```python
from build123d import *

# Parameters (mm, degrees)
SKETCH2_W            = 12
SKETCH2_H            = 29.7
BOSS_EXTRUDE1_DEPTH  = 7.8
SKETCH3_W            = 12
SKETCH3_H            = 2.2
BOSS_EXTRUDE2_DEPTH  = 5.5
CUT_EXTRUDE1_REACH   = 23.628
SKETCH4_R            = 2.35
FILLET1_R            = 1.5
FILLET1_OF_MIRROR1_R = 1.5
FILLET2_R            = 1
BOSS_EXTRUDE3_DEPTH  = 3.2
BOSS_EXTRUDE4_DEPTH  = 0.4
BOSS_EXTRUDE7_DEPTH  = 0.4
SKETCH8_R            = 1.2
BOSS_EXTRUDE6_DEPTH  = 0.2
BOSS_EXTRUDE6_TAPER  = 30
SKETCH7_R            = 2.85
BOSS_EXTRUDE5_DEPTH  = 3.4
SKETCH9_W            = 9
SKETCH9_H            = 5.6
CUT_EXTRUDE2_DEPTH   = 0.1
SKETCH10_R           = 1.1
CUT_EXTRUDE3_DEPTH   = 3
SKETCH13_R           = 4.3
BOSS_EXTRUDE8_DEPTH  = 0.4
FILLET3_R            = 0.4
CUT_EXTRUDE4_DEPTH   = 25.276789326
CIRPATTERN1_COUNT    = 23


with BuildPart() as part:
    # Sketch2 → Boss-Extrude1 (new body)
    with BuildSketch(Plane(origin=(0, 0, 0), x_dir=(1, 0, 0), z_dir=(0, 1, 0))):
        Rectangle(SKETCH2_W, SKETCH2_H)
    extrude(amount=BOSS_EXTRUDE1_DEPTH)

    # Sketch3 → Boss-Extrude2 (add)
    with BuildSketch(Plane.XY.offset(14.85)):
        with Locations((0, 3.1)):
            Rectangle(SKETCH3_W, SKETCH3_H)
    boss_extrude2 = extrude(amount=BOSS_EXTRUDE2_DEPTH)

    # Sketch4 → Cut-Extrude1 (cut, up to next)
    with BuildSketch(Plane(origin=(0, 4.2, 0), x_dir=(1, 0, 0), z_dir=(0, 1, 0)), mode=Mode.PRIVATE) as cut_extrude1_sk1:
        with Locations((0, -18.4)):
            Circle(SKETCH4_R)
    cut_extrude1_tool1 = extrude(cut_extrude1_sk1.sketch, amount=-CUT_EXTRUDE1_REACH, mode=Mode.PRIVATE) & part.part
    cut_extrude1 = cut_extrude1_tool1.solids().sort_by_distance((0, 4.2, 18.4))[0]
    add(cut_extrude1, mode=Mode.SUBTRACT)

    # Fillet1
    fillet1_edges = [part.edges().sort_by_distance(p)[0] for p in [
        (6, 3.1, 20.35),
        (-6, 3.1, 20.35),
    ]]
    fillet(fillet1_edges, radius=FILLET1_R)

    # Mirror1: Boss-Extrude2, Cut-Extrude1 across plane
    add(boss_extrude2.mirror(Plane.XY))
    add(cut_extrude1.mirror(Plane.XY), mode=Mode.SUBTRACT)

    # Fillet1 of Mirror1
    fillet1_of_mirror1_edges = [part.edges().sort_by_distance(p)[0] for p in [
        (6, 3.1, -20.35),
        (-6, 3.1, -20.35),
    ]]
    fillet(fillet1_of_mirror1_edges, radius=FILLET1_OF_MIRROR1_R)

    # Fillet2
    fillet2_edges = [part.edges().sort_by_distance(p)[0] for p in [
        (6, 1, 14.85),
        (6, 6, 14.85),
        (-6, 1, 14.85),
        (-6, 6, 14.85),
        (6, 1, -14.85),
        (6, 6, -14.85),
        (-6, 6, -14.85),
        (-6, 1, -14.85),
    ]]
    fillet(fillet2_edges, radius=FILLET2_R)

    # Sketch5 → Boss-Extrude3 (add)
    with BuildSketch(Plane(origin=(0, 7.8, 0), x_dir=(1, 0, 0), z_dir=(0, 1, 0))):
        with BuildLine():
            Line((-6, 9.155551275), (-6, 1.944448725))
            ThreePointArc((-6, 1.944448725), (-5.292143556, 0.968164496), (-4.427230154, 0.127857143))
            ThreePointArc((-4.427230154, 0.127857143), (0, -6.15), (4.427230154, 0.127857143))
            ThreePointArc((4.427230154, 0.127857143), (5.292143556, 0.968164496), (6, 1.944448725))
            Line((6, 1.944448725), (6, 9.155551275))
            ThreePointArc((6, 9.155551275), (0, 12.55), (-6, 9.155551275))
        make_face()
    extrude(amount=BOSS_EXTRUDE3_DEPTH)

    # Sketch6 → Boss-Extrude4 (add)
    with BuildSketch(Plane(origin=(0, 11, 0), x_dir=(1, 0, 0), z_dir=(0, 1, 0))):
        with BuildLine():
            Line((5.6, 2.057150161), (5.6, 9.042849839))
            ThreePointArc((5.6, 9.042849839), (0, 12.15), (-5.6, 9.042849839))
            Line((-5.6, 9.042849839), (-5.6, 2.057150161))
            ThreePointArc((-5.6, 2.057150161), (-4.856753194, 1.081001408), (-3.945673877, 0.259285714))
            ThreePointArc((-3.945673877, 0.259285714), (0, -5.75), (3.945673877, 0.259285714))
            ThreePointArc((3.945673877, 0.259285714), (4.856753194, 1.081001408), (5.6, 2.057150161))
        make_face()
    extrude(amount=BOSS_EXTRUDE4_DEPTH)

    # Sketch11 → Boss-Extrude7 (add)
    with BuildSketch(Plane(origin=(0, 7.8, 0), x_dir=(1, 0, 0), z_dir=(0, 1, 0))):
        with BuildLine():
            Line((-5.6, 13.85), (-5.6, -13.85))
            ThreePointArc((-5.6, -13.85), (-5.424264069, -14.274264069), (-5, -14.45))
            Line((-5, -14.45), (5, -14.45))
            ThreePointArc((5, -14.45), (5.424264069, -14.274264069), (5.6, -13.85))
            Line((5.6, -13.85), (5.6, 13.85))
            ThreePointArc((5.6, 13.85), (5.424264069, 14.274264069), (5, 14.45))
            Line((5, 14.45), (-5, 14.45))
            ThreePointArc((-5, 14.45), (-5.424264069, 14.274264069), (-5.6, 13.85))
        make_face()
    extrude(amount=BOSS_EXTRUDE7_DEPTH)

    # Sketch8 → Boss-Extrude6 (add)
    with BuildSketch(Plane(origin=(0, 11.4, 0), x_dir=(1, 0, 0), z_dir=(0, 1, 0))):
        with Locations((0, -1.45)):
            Circle(SKETCH8_R)
    extrude(amount=BOSS_EXTRUDE6_DEPTH, taper=BOSS_EXTRUDE6_TAPER)

    # Sketch7 → Boss-Extrude5 (add)
    with BuildSketch(Plane(origin=(0, 11.4, 0), x_dir=(1, 0, 0), z_dir=(0, 1, 0))):
        with Locations(Location((0, 5.55, 0), (0, 0, 270))):
            Circle(SKETCH7_R)
    extrude(amount=BOSS_EXTRUDE5_DEPTH)

    # Sketch9 → Cut-Extrude2 (cut)
    with BuildSketch(Plane(origin=(0, 8.2, 0), x_dir=(1, 0, 0), z_dir=(0, 1, 0))):
        with Locations((0, -10.55)):
            Rectangle(SKETCH9_W, SKETCH9_H)
    extrude(amount=-CUT_EXTRUDE2_DEPTH, mode=Mode.SUBTRACT)

    # Sketch10 → Cut-Extrude3 (cut)
    with BuildSketch(Plane(origin=(0, 14.8, 0), x_dir=(1, 0, 0), z_dir=(0, 1, 0))):
        with Locations(Location((0, 5.55, 0), (0, 0, 270))):
            Circle(SKETCH10_R)
    extrude(amount=-CUT_EXTRUDE3_DEPTH, mode=Mode.SUBTRACT)

    # Sketch13 → Boss-Extrude8 (add)
    with BuildSketch(Plane(origin=(0, 11.4, 0), x_dir=(1, 0, 0), z_dir=(0, 1, 0))):
        with Locations(Location((0, 5.55, 0), (0, 0, 270))):
            Circle(SKETCH13_R)
    extrude(amount=BOSS_EXTRUDE8_DEPTH)

    # Fillet3
    fillet3_edges = [part.edges().sort_by_distance(p)[0] for p in [
        (0, 11.8, -9.85),
    ]]
    fillet(fillet3_edges, radius=FILLET3_R - 0.0001)  # a hair under: the kernel refuses the full size

    # Sketch12 → Cut-Extrude4 (cut, through all)
    with BuildSketch(Plane(origin=(0, 11.8, 0), x_dir=(1, 0, 0), z_dir=(0, 1, 0))):
        Polygon((0, 8.010177118), (-0.466249863, 8.476426981), (0.466249863, 8.476426981), align=None)
    cut_extrude4 = extrude(amount=CUT_EXTRUDE4_DEPTH, mode=Mode.SUBTRACT)

    # CirPattern1: Cut-Extrude4 ×23 about axis
    cirpattern1_axis = Axis((0, 0, -5.55), (0, 1, 0))
    for i in range(1, CIRPATTERN1_COUNT):
        add(cut_extrude4.rotate(cirpattern1_axis, i * 360 / CIRPATTERN1_COUNT), mode=Mode.SUBTRACT)


solid = part.part
```
CAD build for the part. Positions are in the model's coordinates, mm. A direction names the side the tool comes from. Coordinates: 2 decimals unless noted, no trailing zeros. Order: outer loops, then holes, each group sorted by start corner. A loop starts at its lowest first (then second) coordinate and runs counter-clockwise, first axis right, second up. Notation, with made-up numbers: (-14, -6) - (27, -6) arc R6 ccw to (27, -2) - close; hole circle Ø7 at (-5.5, 85). An arc over 180 degrees is marked (long way). Use a Markdown table: item, result. Add a question column.
(1) Saw through at B-B (y = 2.75). Give the cut face in (x, z), then the cut area to 3 significant figures.
(2) Pull direction Z, two halves, no side cores. Call faces 4 (the face through (-0.12, 11.2, 5.75)), 5 (the face through (0, 1, 14.85)), 6 (the face through (5.57, 3.12, -19.9)), 7 (the face through (-6, 4, 0)): +Z half, -Z half, draft (parallel to the pull), parting line (faces both ways), or undercut.
(3) Which spindle directions (+Z, -Z, +X, -X, +Y, -Y) get a long thin tool onto all of the face, cutting with end or side? Do faces 1 (the face through (5.699, 6.025, -14.565)), 2 (the face through (-1, 11.4, -1)), 3 (the face through (0, 6, -14.85)). Say none if no direction does.
(4) Saw through at C-C (z = 7). Give the cut face in (x, y), then the cut area to 3 significant figures.
(5) Saw through at A-A (z = -18.4). Give the cut face in (x, y).
(6) Flat gauge pins, fed straight in: pin 1 (2 mm diameter, centred on x = 0.5, z = 16, fed in from -Y); pin 2 (3.5 mm diameter, centred on x = 2.5, z = 18, fed in from +Y); pin 3 (3 mm diameter, centred on x = -3.5, y = 13, fed in from -Z); pin 4 (5 mm diameter, centred on x = 1.5, z = 8, fed in from -Y). Where does each tip first touch, or does it go through?
(7) Drill centre lines: line 1 along X through (y, z) = (3.1, -18.4); line 2 along Y through (x, z) = (0.75, -15); line 3 along Y through (x, z) = (3, -10.5). Where is each one in solid material? Low to high. Write a range as [from, to].
Solved:
| question | item | result |
|---|---|---|
| 1 | outline | (-6, -18.85) arc R1.5 ccw to (-4.5, -20.35) - (-1.31, -20.35) arc R2.35 cw (long way) to (1.31, -20.35) - (4.5, -20.35) arc R1.5 ccw to (6, -18.85) - (6, 18.85) arc R1.5 ccw to (4.5, 20.35) - (1.31, 20.35) arc R2.35 cw (long way) to (-1.31, 20.35) - (-4.5, 20.35) arc R1.5 ccw to (-6, 18.85) - close |
| 1 | area | 453 mm² |
| 2 | face 4 | undercut |
| 2 | face 5 | +Z half |
| 2 | face 6 | -Z half |
| 2 | face 7 | draft |
| 3 | face 1 | -Z, +X, +Y |
| 3 | face 2 | +Y |
| 3 | face 3 | -Z, +X, -X, +Y |
| 4 | outline | (-6, 0) - (6, 0) - (6, 7.8) - (5.6, 7.8) - (5.6, 8.2) - (-5.6, 8.2) - (-5.6, 7.8) - (-6, 7.8) - close |
| 4 | area | 98.1 mm² |
| 5 | outline | (-6, 2) - (-2.35, 2) - (-2.35, 4.2) - (-6, 4.2) - close; (2.35, 2) - (6, 2) - (6, 4.2) - (2.35, 4.2) - close |
| 6 | pin 1 | stops at y = 2 |
| 6 | pin 2 | stops at y = 4.2 |
| 6 | pin 3 | stops at z = -8.68 |
| 6 | pin 4 | stops at y = 0 |
| 7 | line 1 | x = [-6, -2.35], [2.35, 6] |
| 7 | line 2 | y = [2, 4.2] |
| 7 | line 3 | y = [0, 11.4] |
